Here's the drawing with two shaded views (mm, measured from the low corner). I have some questions. A direction names the side the tool comes from. Coordinates: 2 decimals unless noted, no trailing zeros. Order: outer loops, then holes, each group sorted by start corner. A loop starts at its lowest first (then second) coordinate and runs counter-clockwise, first axis right, second up. Notation, with made-up numbers: (40, 43.5) - (92, 43.5) arc R35 cw to (92, 76.5) - close; hole circle Ø10 at (-10.75, 55.25). An arc over 180 degrees is marked (long way). Answer as a JSON object with one key per item and string values. Group by question number.
(1) Will these pins go through, and if not, where does the flat tip stop? P1, Ø12, axis at x = 7.5, y = 57, coming from the -Z side; P2, Ø10, axis at x = 6, y = 52.5, coming from the +Z side; P3, Ø4, axis at x = 3.5, z = 5.5, coming from the -Y side; P4, Ø3, axis at x = 22, z = 8.5, coming from the +Y side.
(2) Imagine slicing it at C-C, the plane y = 49.5. Write out the boundary of the cut face in (x, z), and give its area (3 significant figures).
(3) Which directions (+Z, -Z, +X, -X, +Y, -Y) give clear straight access to the entire face, cutting with the end or side of a thin tool? Please do the marked faces 1 and 2.
(4) Imagine slicing it at A-A, the plane z = 12.5. Write out the boundary of the cut face in (x, y) (3 decimals).
(5) Imagine slicing it at D-D, the plane z = 20.25. Write out the boundary of the cut face in (x, y).
(6) Imagine slicing it at B-B, the plane y = 6.5. Write out the boundary of the cut face in (x, z), and give its area (3 significant figures).
(7) Please list where these lines run through material, in increasing order: probe 1 along Y at (x, z) = (7.25, 7); probe 2 along Y at (x, z) = (11.25, 18); probe 3 along Z at (x, y) = (15.5, 42.5).
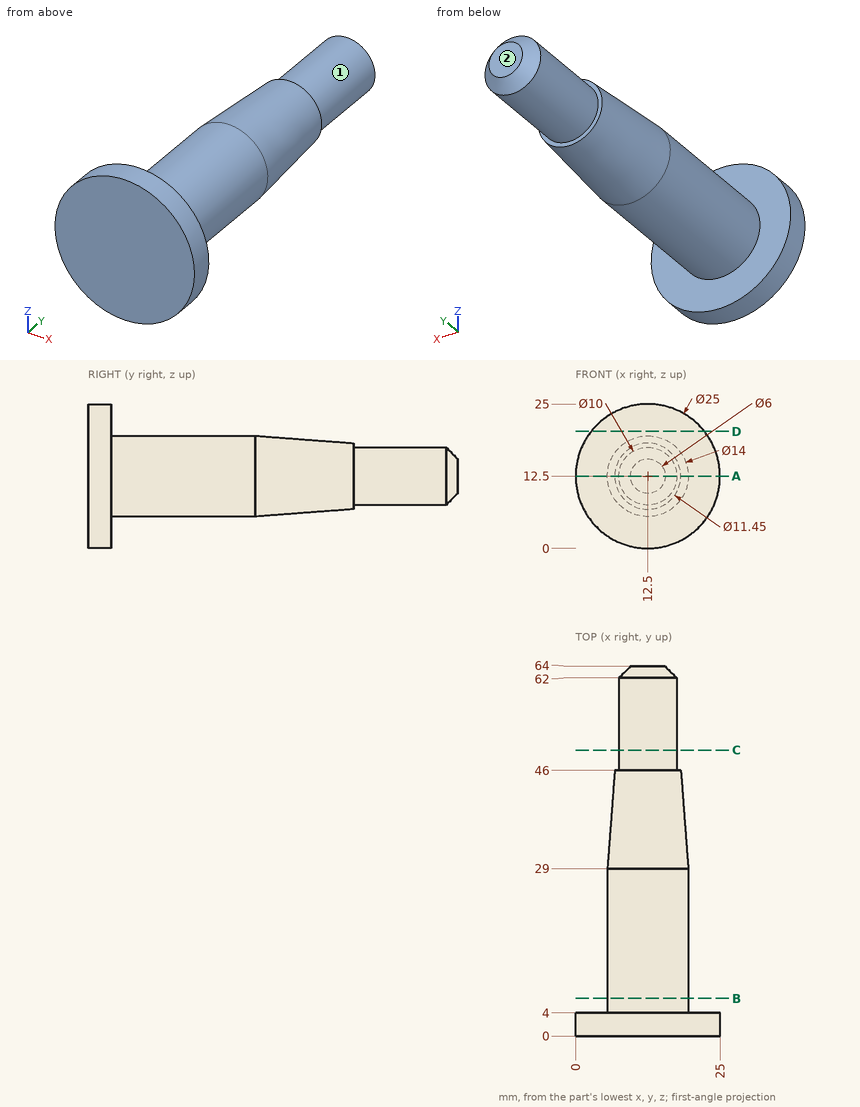
Result set:
{
 "1": {"P1": "stops at z = 7.5", "P2": "stops at z = 17.27", "P3": "stops at y = 0", "P4": "stops at y = 4"},
 "2": {"outline": "circle Ø10 at (12.5, 12.5)", "area": "78.5 mm^2"},
 "3": {"face 1": "+Y", "face 2": "+Z, -Z, +X, -X, +Y"},
 "4": {"outline": "(0, 0) - (25, 0) - (25, 4) - (19.5, 4) - (19.5, 29) - (18.225, 46) - (17.5, 46) - (17.5, 62) - (15.5, 64) - (9.5, 64) - (7.5, 62) - (7.5, 46) - (6.775, 46) - (5.5, 29) - (5.5, 4) - (0, 4) - close"},
 "5": {"outline": "(2.69, 0) - (22.31, 0) - (22.31, 4) - (2.69, 4) - close"},
 "6": {"outline": "circle Ø14 at (12.5, 12.5)", "area": "154 mm^2"},
 "7": {"probe 1": "y = 0 to 4", "probe 2": "y = 0 to 46", "probe 3": "z = 7.32 to 17.68"}
}
